Read the model definition and answer for the solid it produces. Units are mm, in the model's axes. A direction names the side the tool comes from. Coordinates: 2 decimals unless noted, no trailing zeros.
```python
from build123d import *

# Parameters (mm, degrees)
SKETCH_W        = 102
SKETCH_H        = 102
PAD_DEPTH       = 2
SKETCH001_R     = 17.7
SKETCH001_R_2   = 1.5
SKETCH001_W     = 10
SKETCH001_H     = 2.4
SKETCH001_W_2   = 2.4
SKETCH001_H_2   = 10
POCKET_DEPTH    = 2.001
SKETCH002_R     = 4
SKETCH002_R_2   = 1.15
PAD001_DEPTH    = 7.7
SKETCH003_W     = 20
SKETCH003_H     = 2
SKETCH003_W_2   = 2
SKETCH003_H_2   = 20
PAD002_DEPTH    = 20
SKETCH004_W     = 55
SKETCH004_H     = 40
SKETCH004_W_2   = 51
SKETCH004_H_2   = 36
PAD003_DEPTH    = 4
SKETCH005_W     = 2
SKETCH005_H     = 29
SKETCH005_W_2   = 21.5
SKETCH005_H_2   = 2
PAD004_DEPTH    = 3
POCKET001_DEPTH = 2.001
FILLET_R        = 15


with BuildPart() as part:
    # Sketch → Pad (new body)
    with BuildSketch(Plane.XY):
        Rectangle(SKETCH_W, SKETCH_H)
    extrude(amount=PAD_DEPTH)

    # Sketch001 → Pocket (cut, through all)
    with BuildSketch(Plane.XY.offset(2)):
        Circle(SKETCH001_R)
        with Locations((-21, 0)):
            Circle(SKETCH001_R_2)
        with Locations((21, 0)):
            Circle(SKETCH001_R_2)
        with Locations((-15, 46.6)):
            Rectangle(SKETCH001_W, SKETCH001_H)
        with Locations((15, 46.6)):
            Rectangle(SKETCH001_W, SKETCH001_H)
        with Locations((46.6, 15)):
            Rectangle(SKETCH001_W_2, SKETCH001_H_2)
        with Locations((46.6, -15)):
            Rectangle(SKETCH001_W_2, SKETCH001_H_2)
        with Locations((15, -46.6)):
            Rectangle(SKETCH001_W, SKETCH001_H)
        with Locations((-15, -46.6)):
            Rectangle(SKETCH001_W, SKETCH001_H)
        with Locations((-46.6, 15)):
            Rectangle(SKETCH001_W_2, SKETCH001_H_2)
        with Locations((-46.6, -15)):
            Rectangle(SKETCH001_W_2, SKETCH001_H_2)
    extrude(amount=-POCKET_DEPTH, mode=Mode.SUBTRACT)

    # Sketch002 → Pad001 (new body)
    with BuildSketch(Plane.XY.offset(2)):
        with Locations((15.45, -27.6)):
            Circle(SKETCH002_R)
        with Locations((15.45, -27.6)):
            Circle(SKETCH002_R_2, mode=Mode.SUBTRACT)
        with Locations((-8.7, -31.3)):
            Circle(SKETCH002_R)
        with Locations((-8.7, -31.3)):
            Circle(SKETCH002_R_2, mode=Mode.SUBTRACT)
    extrude(amount=PAD001_DEPTH)

    # Sketch003 → Pad002 (new body)
    with BuildSketch(Plane.XY.offset(2)):
        Polygon((-51, 36), (-49, 36), (-49, 49), (-36, 49), (-36, 51), (-51, 51), align=None)
        Polygon((36, 51), (36, 49), (49, 49), (49, 36), (51, 36), (51, 51), align=None)
        Polygon((51, -36), (51, -51), (36, -51), (36, -49), (49, -49), (49, -36), align=None)
        Polygon((-51, -51), (-36, -51), (-36, -49), (-49, -49), (-49, -36), (-51, -36), align=None)
        with Locations((0, 50)):
            Rectangle(SKETCH003_W, SKETCH003_H)
        with Locations((50, 0)):
            Rectangle(SKETCH003_W_2, SKETCH003_H_2)
        with Locations((0, -50)):
            Rectangle(SKETCH003_W, SKETCH003_H)
        with Locations((-50, 0)):
            Rectangle(SKETCH003_W_2, SKETCH003_H_2)
    extrude(amount=PAD002_DEPTH)

    # Sketch004 → Pad003 (new body)
    with BuildSketch(Plane.XY.offset(2)):
        Rectangle(SKETCH004_W, SKETCH004_H)
        Rectangle(SKETCH004_W_2, SKETCH004_H_2, mode=Mode.SUBTRACT)
    extrude(amount=PAD003_DEPTH)

    # Sketch005 → Pad004 (new body)
    with BuildSketch(Plane.XY.offset(2)):
        with Locations((0, 34.5)):
            Rectangle(SKETCH005_W, SKETCH005_H)
        with Locations((38.25, 0)):
            Rectangle(SKETCH005_W_2, SKETCH005_H_2)
        with Locations((0, -34.5)):
            Rectangle(SKETCH005_W, SKETCH005_H)
        with Locations((-38.25, 0)):
            Rectangle(SKETCH005_W_2, SKETCH005_H_2)
        Polygon((-27.5, 18.808883), (-49, 47.808883), (-49, 49), (-47.393376, 49), (-25.893376, 20), (-27.5, 20), align=None)
        Polygon((25.893376, 20), (47.393376, 49), (49, 49), (49, 47.808883), (27.5, 18.808883), (27.5, 20), align=None)
        Polygon((47.393376, -49), (25.893376, -20), (27.5, -20), (27.5, -18.808883), (49, -47.808883), (49, -49), align=None)
        Polygon((-47.393376, -49), (-49, -49), (-49, -47.808883), (-27.5, -18.808883), (-27.5, -20), (-25.893376, -20), align=None)
    extrude(amount=PAD004_DEPTH)

    # Sketch006 → Pocket001 (cut, through all)
    with BuildSketch(Plane.XY.offset(2)):
        Polygon((-41.925284, 46.487865), (-23.968742, 22.569384), (-4.320471, 22.569384), (-4.320471, 43.105819), (-22.587998, 43.105819), (-22.587998, 46.487865), align=None)
        Polygon((2.93549, 41.811786), (2.93549, 22.665701), (24.092464, 22.665701), (41.469131, 46.201939), (24.769491, 46.201939), (24.769491, 41.811786), align=None)
        Polygon((46.52763, 38.437729), (46.52763, 22.923718), (43.001148, 22.923718), (43.001148, 3.595317), (30.999222, 3.595317), (30.999222, 17.497902), align=None)
        Polygon((46.533894, -38.494362), (46.533894, -23.565529), (42.681282, -23.565529), (42.681282, -3.724627), (29.967691, -3.724627), (29.967691, -17.593996), align=None)
        Polygon((40.177086, -46.199566), (24.188789, -46.199566), (24.188789, -42.924854), (5.40735, -42.924854), (5.40735, -35.412281), (23.610897, -35.412281), (23.610897, -25.010254), align=None)
        Polygon((-39.860725, -45.910622), (-25.124525, -25.395514), (-16.745111, -25.395514), (-16.745111, -41.865391), (-22.235073, -41.865391), (-22.235073, -45.910622), align=None)
        Polygon((-46.410149, 36.92033), (-46.410149, 24.206741), (-41.787029, 24.206741), (-41.787029, 5.232674), (-30.710796, 5.232674), (-30.710796, 18.71678), align=None)
        Polygon((-46.699104, -39.072254), (-46.699104, -23.276583), (-41.112823, -23.276583), (-41.112823, -4.206202), (-30.999743, -4.206202), (-30.999743, -18.2682), align=None)
    extrude(amount=-POCKET001_DEPTH, mode=Mode.SUBTRACT)

    # Fillet
    fillet_edges = [part.edges().sort_by_distance(p)[0] for p in [
        (-49, 0, 5),
        (0, 49, 5),
        (49, 0, 5),
        (0, -49, 5),
    ]]
    fillet(fillet_edges, radius=FILLET_R)


solid = part.part
```
1) A flat-ended cylindrical pin translates along its axis: pin 1 Ø8 at (x, y) = (26, 41) entering from +Z. Find the tip coordinate at first contact, or state that the pin passes through.
A:
pin 1: stops at z = 2
2) Determine the mould class of faces 4 (the flat face through (1, 51, 8)), 5 (the flat face through (31.78, -35.46, 1.01)), 6 (the flat face through (51, -1, 8)) for opening direction X: pulls with the +X half, pulls with the -X half, needs draft (parallel to the pull), parting line crosses it, or undercut.
A:
face 4: needs draft
face 5: undercut
face 6: pulls with the +X half
3) A cutting plane is placed at A-A, the plane y = 14.5. State how many separate pieces and enclosed holes the cut face has, and give its area (3 significant figures).
A:
separate pieces: 6
enclosed holes: 0
area: 124 mm2
4) Straight lines are drawn through the part: line 1 (Y direction, x = 21, z = 1.4); line 2 (X direction, y = 2, z = 3.25); line 3 (Y direction, x = 7, z = 3.25). For each, find the intervals that lie inside material, in ascending order.
A:
line 1: y = -51 to -42.92, -35.41 to -1.5, 1.5 to 22.67, 41.81 to 51
line 2: x = -51 to -49, -27.5 to -25.5, 25.5 to 27.5, 49 to 51
line 3: y = -51 to -49, -20 to -18, 18 to 20, 49 to 51
5) Which of the six approach directions +Z, -Z, +X, -X, +Y, -Y give full straight-line access (tool end or side, diameter ignored) to faces 1 (the flat face through (38.655, 27.821, 1.014)), 2 (the flat face through (-46, 50, 22)), 3 (the flat face through (-49, -43, 12))?
A:
face 1: +Z, -Z
face 2: +Z, +X, -X, +Y, -Y
face 3: +Z
